Answer from the drawing. Dimensions are ordinates in mm from the lowest x, y and z of the part. A direction names the side the tool comes from. Give positions to 0.01 mm unless a question says otherwise; leave off trailing zeros. Write each loop counter-clockwise with the first axis right and the second up, starting at its lowest first coordinate (ties: lowest second). Pieces come first, ordered by that corner, then holes. Notation, with made-up numbers: (29.25, 86.25) -> (57.25, 86.25) arc R22 ccw to (57.25, 116.25) -> close; hole circle Ø4 at (-27, -15.75). An arc over 180 degrees is marked (long way). Put each result on its own line as item: value. Start each with the question number.
1) For a pull along X with two mould halves and no side action, classify the marked faces 1, 2 and 3 as released by +X, released by -X, zero draft, split by the parting line, or undercut.
2) Flat-ended cylindrical pins translate along their axes: pin 1 Ø1.6 at (x, z) = (33.5, 1.5) entering from -Y; pin 2 Ø1.6 at (x, z) = (3, 1) entering from +Y; pin 3 Ø1 at (y, z) = (3, 2) entering from +X. Find the tip coordinate at first contact, or state that the pin passes through.
3) A cutting plane is placed at A-A (y = 12.75). Write down the section's boundary in (x, z) (1 decimal).
4) Find the intervals of material crossed by line 1 along X through (y, z) = (3, 2) (1 decimal); line 2 along Y through (x, z) = (12, 0.25), in increasing order. Write a range as from..to.
5) A cutting plane is placed at B-B (z = 0.7). Write down the section's boundary in (x, y) (1 decimal).
6) For the marked faces 4, 5, 6, 7 and 8, determine the directions among +Z, -Z, +X, -X, +Y, -Y from which every point of the face is accessible in a straight line to the end or side of a thin tool.
7) A cutting plane is placed at C-C (x = 12.5). Write down the section's boundary in (y, z) (1 decimal).
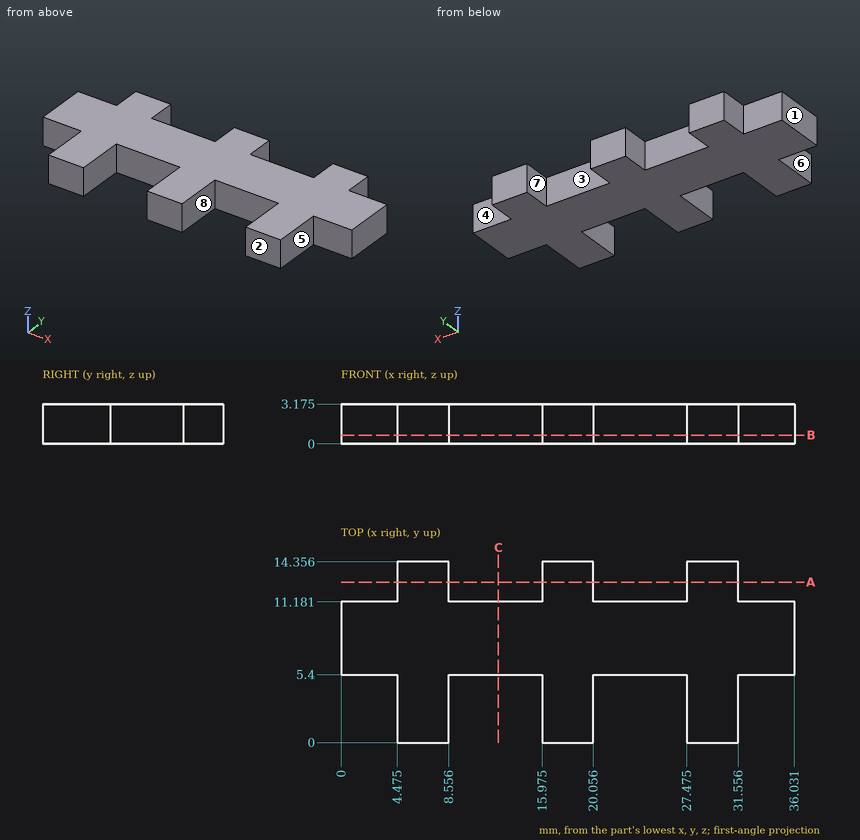
Reply:
1. face 1: released by -X
1. face 2: zero draft
1. face 3: undercut
2. pin 1: stops at y = 5.4
2. pin 2: stops at y = 11.18
2. pin 3: stops at x = 31.56
3. outline: (4.5, 0) -> (8.6, 0) -> (8.6, 3.2) -> (4.5, 3.2) -> close; (16, 0) -> (20.1, 0) -> (20.1, 3.2) -> (16, 3.2) -> close; (27.5, 0) -> (31.6, 0) -> (31.6, 3.2) -> (27.5, 3.2) -> close
4. line 1: x = 4.5..8.6, 16..20.1, 27.5..31.6
4. line 2: y = 5.4..11.18
5. outline: (0, 5.4) -> (4.5, 5.4) -> (4.5, 0) -> (8.6, 0) -> (8.6, 5.4) -> (16, 5.4) -> (16, 0) -> (20.1, 0) -> (20.1, 5.4) -> (27.5, 5.4) -> (27.5, 0) -> (31.6, 0) -> (31.6, 5.4) -> (36, 5.4) -> (36, 11.2) -> (31.6, 11.2) -> (31.6, 14.4) -> (27.5, 14.4) -> (27.5, 11.2) -> (20.1, 11.2) -> (20.1, 14.4) -> (16, 14.4) -> (16, 11.2) -> (8.6, 11.2) -> (8.6, 14.4) -> (4.5, 14.4) -> (4.5, 11.2) -> (0, 11.2) -> close
6. face 4: +Z, -Z, +X, +Y
6. face 5: +Z, -Z, +X, -Y
6. face 6: +Z, -Z, -X, -Y
6. face 7: +Z, -Z, +Y
6. face 8: +Z, -Z, -Y
7. outline: (5.4, 0) -> (11.2, 0) -> (11.2, 3.2) -> (5.4, 3.2) -> close
